Here's how the part is built. I have some questions about the finished solid (model axes, mm). A direction names the side the tool comes from. Coordinates: 2 decimals unless noted, no trailing zeros. Write each loop counter-clockwise with the first axis right and the second up, starting at its lowest first coordinate (ties: lowest second). Pieces come first, ordered by that corner, then holes.
from build123d import *

# Parameters (mm, degrees)
SKETCH1_R               = 6
BOSS_EXTRUDE1_DEPTH     = 10
CUT_EXTRUDE1_REACH      = 15.115
CUT_EXTRUDE1_END_RADIUS = 6
SKETCH3_R               = 1.5
SKETCH4_R               = 6
BOSS_EXTRUDE2_DEPTH     = 2
BOSS_EXTRUDE3_DEPTH     = 10
CHAMFER1_SIZE           = 0.75
CIRPATTERN1_COUNT       = 3


with BuildPart() as part:
    # Sketch1 → Boss-Extrude1 (new body)
    with BuildSketch(Plane.XY):
        Circle(SKETCH1_R)
        with BuildLine():
            Line((-1.598436736, 1.475), (1.598436736, 1.475))
            ThreePointArc((1.598436736, 1.475), (0, -2.175), (-1.598436736, 1.475))
        make_face(mode=Mode.SUBTRACT)
    extrude(amount=BOSS_EXTRUDE1_DEPTH)

    # Cut-Extrude1: up to this cylinder (the profile starts inside it)
    cut_extrude1_end = Plane(origin=(0, 0, 5), z_dir=(0, 0, -1)) * Cylinder(CUT_EXTRUDE1_END_RADIUS, 47.23, mode=Mode.PRIVATE)
    # Sketch3 → Cut-Extrude1 (cut, up to the surface)
    with BuildSketch(Plane(origin=(0, 0, 0), x_dir=(1, 0, 0), z_dir=(0, 1, 0)), mode=Mode.PRIVATE) as cut_extrude1_sk1:
        with Locations(Location((0, -3, 0), (0, 0, 90))):
            Circle(SKETCH3_R)
    cut_extrude1_tool1 = extrude(cut_extrude1_sk1.sketch, amount=CUT_EXTRUDE1_REACH, mode=Mode.PRIVATE) & cut_extrude1_end
    # Sketch3 → Cut-Extrude1 (cut, up to the surface)
    with BuildSketch(Plane(origin=(0, 0, 0), x_dir=(1, 0, 0), z_dir=(0, 1, 0)), mode=Mode.PRIVATE) as cut_extrude1_sk2:
        with Locations(Location((0, -7, 0), (0, 0, 90))):
            Circle(SKETCH3_R)
    cut_extrude1_tool2 = extrude(cut_extrude1_sk2.sketch, amount=CUT_EXTRUDE1_REACH, mode=Mode.PRIVATE) & cut_extrude1_end
    cut_extrude1 = cut_extrude1_tool1.solids().sort_by_distance((0, 0, 3))[0] + cut_extrude1_tool2.solids().sort_by_distance((0, 0, 7))[0]
    add(cut_extrude1, mode=Mode.SUBTRACT)

    # Sketch4 → Boss-Extrude2 (add)
    with BuildSketch(Plane.XY.offset(10)):
        Circle(SKETCH4_R)
    extrude(amount=BOSS_EXTRUDE2_DEPTH)

    # Sketch6 → Boss-Extrude3 (add)
    with BuildSketch(Plane.XY.offset(12)):
        with BuildLine():
            Line((2.655183609, 3.025), (-2.655183609, 3.025))
            ThreePointArc((-2.655183609, 3.025), (-1.660348001, -3.666588266), (4.025, 0))
            ThreePointArc((4.025, 0), (3.666588266, 1.660348001), (2.655183609, 3.025))
        make_face()
    extrude(amount=BOSS_EXTRUDE3_DEPTH)

    # Chamfer1
    chamfer1_edges = [part.edges().sort_by_distance(p)[0] for p in [
        (-6, 0, 0),
    ]]
    chamfer(chamfer1_edges, length=CHAMFER1_SIZE)

    # CirPattern1: Cut-Extrude1 ×3 about axis
    cirpattern1_axis = Axis((0, 0, 0), (0, 0, -1))
    for i in range(1, CIRPATTERN1_COUNT):
        add(cut_extrude1.rotate(cirpattern1_axis, i * 360 / CIRPATTERN1_COUNT), mode=Mode.SUBTRACT)


solid = part.part
1. Thinking about a two-plate mould opening in Y: for faces 1 (the face through (-1.301, -5.857, 6.296)), 2 (the face through (0, 1.475, 5)), 3 (the face through (0, 0, 22)), which applies, pulls with the +Y half, pulls with the -Y half, needs draft (parallel to the pull), parting line crosses it, or undercut?
2. I want a section at D-D (y = 3.5). State how many separate pieces and enclosed holes the cut face has, then the cut area to 3 significant figures.
3. On a 3-axis mill with a long thin cutter (end or side, diameter ignored), from which of +Z, -Z, +X, -X, +Y, -Y can I reach the whole of each face in a straight line? I mean faces 4 (the face through (-0.07, 3.71, 8.5)), 5 (the face through (0.071, -2.174, 4.93)), 6 (the face through (0, 3.025, 17)). Say none if no direction works.
4. I want a section at B-B (z = 7). List the corners of the cut face in (x, y) for me (3 decimals).
5. If I drill on line 1 (X direction, y = 2.9, z = 3); line 2 (Z direction, x = 1.5, y = -2.25); line 3 (Z direction, x = 4.75, y = -2.25), over which ranges is the centre line in solid material (lowest first)?
6. I want a section at A-A (x = 0). List the corners of the cut face in (y, z) for me (3 decimals), then the cut area to 3 significant figures.
7. I want a section at C-C (z = 13). List the corners of the cut face in (x, y) for me (3 decimals), then the cut area to 3 significant figures.
8. For pin 1 Ø1.5 at (y, z) = (-4, 17) entering from +X; pin 2 Ø2.5 at (x, z) = (-1, 15) entering from +Y (3 decimals); pin 3 Ø1.8 at (x, y) = (0.5, -0.5) entering from -Z, each with a flat end and sliding along its axis, tell me the tip position at first contact or that it passes through.
Response values:
1. face 1: parting line crosses it
1. face 2: undercut
1. face 3: needs draft
2. separate pieces: 1
2. enclosed holes: 2
2. area: 102 mm2
3. face 4: +Y
3. face 5: -Z
3. face 6: +Z, +X, -X, +Y
4. outline: (-5.781, -1.606) - (-2.114, 0.512) arc R2.175 cw to (-1.598, 1.475) - (-1.5, 1.475) - (-1.5, 5.809) arc R6 ccw to start; (-4.281, -4.204) arc R6 ccw to (4.281, -4.204) - (0.614, -2.087) arc R2.175 cw to (-0.614, -2.087) - close; (1.5, 1.475) - (1.598, 1.475) arc R2.175 cw to (2.114, 0.512) - (5.781, -1.606) arc R6 ccw to (1.5, 5.809) - close
5. line 1: x = -5.25 to -1.5, 1.5 to 5.25
5. line 2: z = 0 to 2.1, 3.9 to 6.1, 7.9 to 22
5. line 3: z = 0.01 to 1.56, 4.44 to 5.56, 8.44 to 12
6. outline: (-6, 0.75) - (-5.25, 0) - (-2.175, 0) - (-2.175, 10) - (1.475, 10) - (1.475, 8.5) - (6, 8.5) - (6, 12) - (3.025, 12) - (3.025, 22) - (-4.025, 22) - (-4.025, 12) - (-6, 12) - close; (1.475, 0) - (5.25, 0) - (6, 0.75) - (6, 1.5) - (1.475, 1.5) - close; (1.475, 4.5) - (6, 4.5) - (6, 5.5) - (1.475, 5.5) - close
6. area: 150 mm2
7. outline: (-2.655, 3.025) arc R4.025 ccw (long way) to (2.655, 3.025) - close
7. area: 47.3 mm2
8. pin 1: stops at x = 2.37
8. pin 2: stops at y = 3.025
8. pin 3: stops at z = 10
